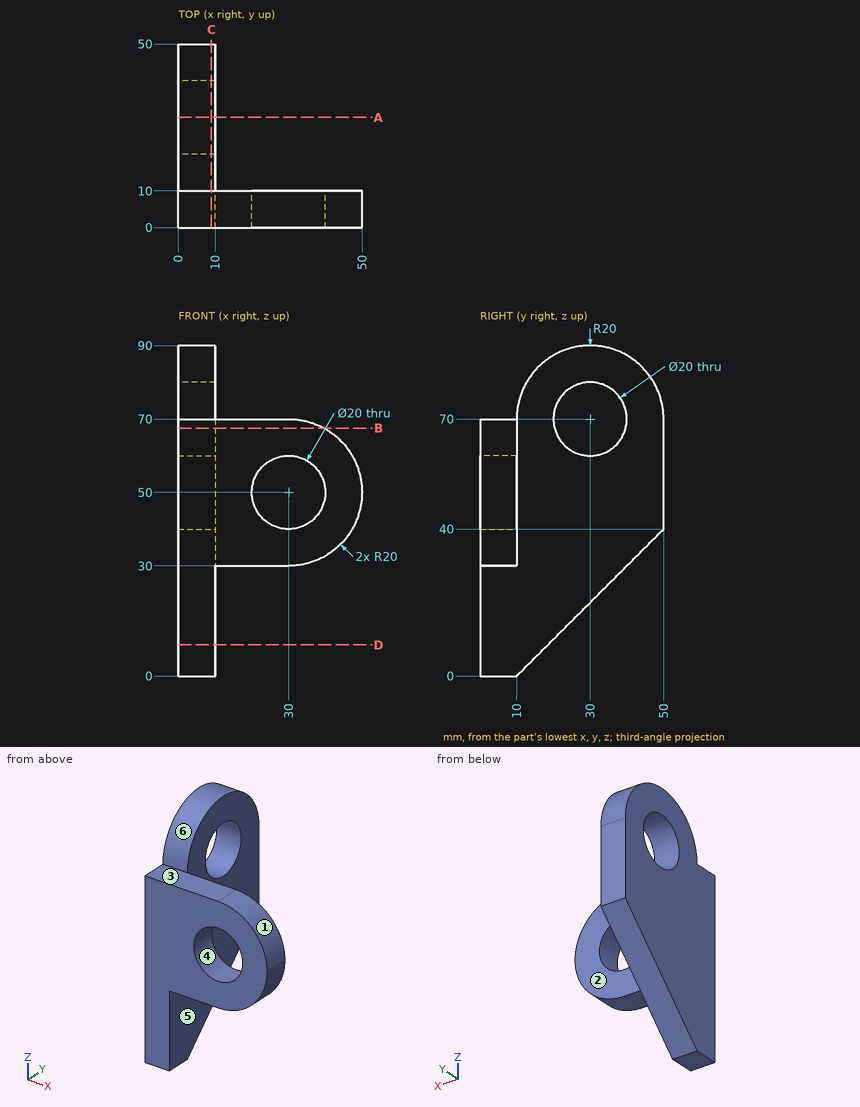
Geometry check sheet. Reference: drawing and pictorial views, mm from the part's lowest x, y, z. A direction names the side the tool comes from. Coordinates: 2 decimals unless noted, no trailing zeros. Write each loop counter-clockwise with the first axis right and the second up, starting at its lowest first coordinate (ties: lowest second). Pieces come first, ordered by that corner, then holes.
Item 1: Scan lines: probe 1 along X at (y, z) = (2, 50); probe 2 along X at (y, z) = (25, 41.5); probe 3 along Z at (x, y) = (13, 9.5). Record each from-to range of solid material in increasing order.
Numbers:
probe 1: x = 0 to 20, 40 to 50
probe 2: x = 0 to 10
probe 3: z = 30 to 70
Item 2: Mould release check, pull along Z, two halves, no side actions. Record for the marked faces 4, 5 and 6: released by +Z, released by -Z, zero draft, split by the parting line, or undercut.
Numbers:
face 4: undercut
face 5: zero draft
face 6: released by +Z
Item 3: Cross-section at D-D on z = 8.5. Record the boundary of the cut face in (x, y).
Numbers:
outline: (0, 0) - (10, 0) - (10, 18.5) - (0, 18.5) - close
Item 4: Cross-section at A-A on y = 30. Record the boundary of the cut face in (x, z), then the cut area to 3 significant figures.
Numbers:
outline: (0, 20) - (10, 20) - (10, 60) - (0, 60) - close; (0, 80) - (10, 80) - (10, 90) - (0, 90) - close
area: 500 mm2
Item 5: Cross-section at C-C on x = 9. Record the boundary of the cut face in (y, z), then the cut area to 3 significant figures.
Numbers:
outline: (0, 0) - (10, 0) - (50, 40) - (50, 70) arc R20 ccw to (10, 70) - (0, 70) - close; hole circle Ø20 at (30, 70)
area: 3,010 mm2
Item 6: Cross-section at B-B on z = 67.5. Record the boundary of the cut face in (x, y), then the cut area to 3 significant figures.
Numbers:
outline: (0, 0) - (39.68, 0) - (39.68, 10) - (10, 10) - (10, 20.32) - (0, 20.32) - close; (0, 39.68) - (10, 39.68) - (10, 50) - (0, 50) - close
area: 603 mm2
Item 7: Access from +Z, -Z, +X, -X, +Y, -Y to the whole of each face (thin tool, end or side, straight path). Record for the marked faces 1, 2 and 3.
Numbers:
face 1: +Z, +X, +Y, -Y
face 2: +Z, -Z, +X, +Y
face 3: +Z, +X, -X, -Y
Item 8: Depth check by flat-ended pin: pin 1 Ø18 at (x, z) = (30, 50) entering from -Y; pin 2 Ø5 at (x, y) = (24.5, 5) entering from -Z; pin 3 Ø20 at (x, z) = (29.5, 58) entering from +Y; pin 4 Ø2 at (y, z) = (25.5, 21) entering from +X. Enter the tip coordinate at first touch or a pass-through.
Numbers:
pin 1: passes through
pin 2: stops at z = 30
pin 3: stops at y = 10
pin 4: stops at x = 10
